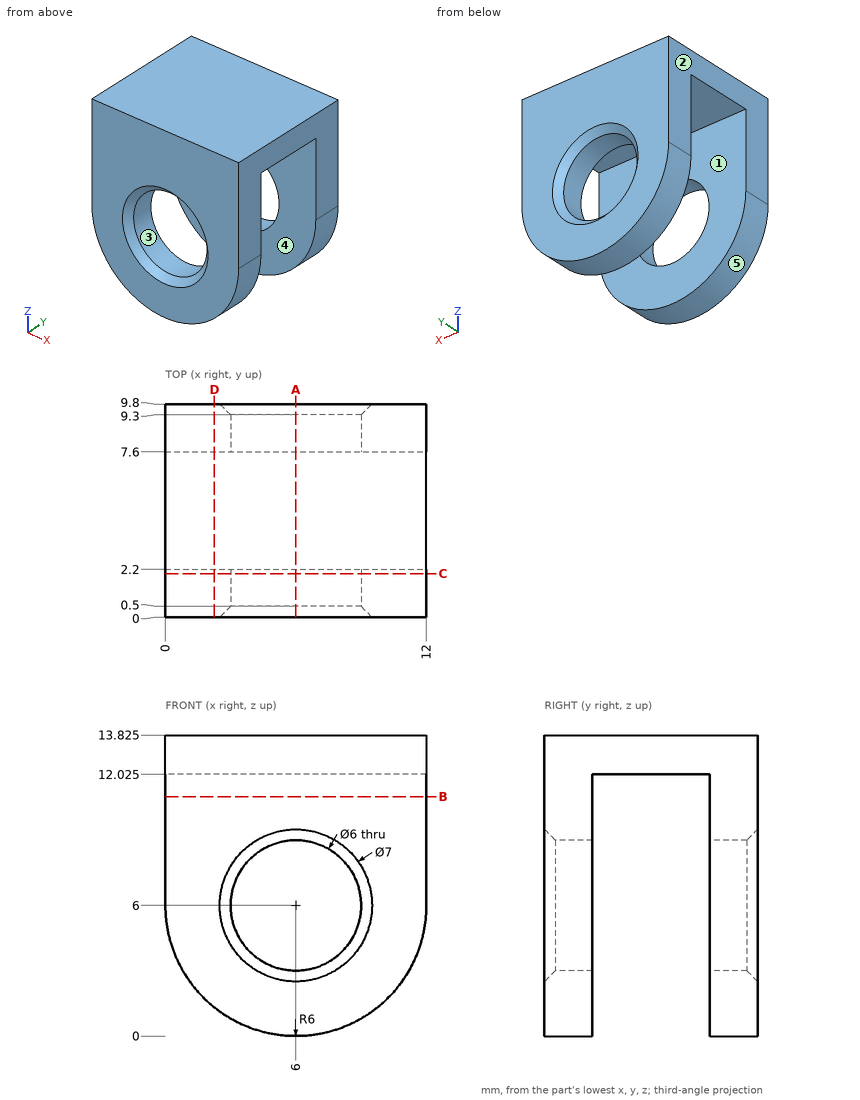
Geometry check sheet. Reference: drawing and pictorial views, mm from the part's lowest x, y, z. A direction names the side the tool comes from. Give positions to 0.01 mm unless a question says otherwise; leave off trailing zeros. Order: outer loops, then holes, each group sorted by start corner. A loop starts at its lowest first (then second) coordinate and runs counter-clockwise, first axis right, second up. Notation, with made-up numbers: M 53,-6 L 82,-6 A25 cw 82,14 Z; hole C 18,78 d8. An arc over 180 degrees is marked long. Use one line per item in the form item = value. Start each with the question number.
Q1. Scan lines: line 1 along Y through (x, z) = (9.25, 2.5); line 2 along X through (y, z) = (8.5, 6); line 3 along Z through (x, y) = (6, 8.75) (3 decimals). Record each from-to range of solid material in increasing order. Write a range as [from, to].
Q2. Access from +Z, -Z, +X, -X, +Y, -Y to the whole of each face (thin tool, end or side, straight path). Record for the marked faces 4 and 5.
Q3. Section check D-D (x = 2.25). Enter the section's corners in (y, z) (3 decimals).
Q4. Go/stop test with flat-tipped pins: pin 1 Ø1.5 at (y, z) = (2, 5) entering from -X; pin 2 Ø4 at (x, y) = (3.5, 3.5) entering from -Z; pin 3 Ø1 at (x, y) = (8.5, 8) entering from -Z. Record where each tip stops, or that it passes through.
Q5. Section check A-A (x = 6). Enter the section's corners in (y, z) (3 decimals).
Q6. Section check C-C (y = 2). Enter the section's corners in (x, z) (3 decimals).
Q7. Mould release check, pull along X, two halves, no side actions. Record for the marked faces 1, 2 and 3: +X half, -X half, draft (parallel to the pull), parting line (faces both ways), or undercut.
Q8. Section check B-B (z = 11). Enter the section's corners in (x, y).
Evaluation:
q1.line_1 = [0, 2.2], [7.6, 9.8]
q1.line_2 = [0, 3], [9, 12]
q1.line_3 = [0, 3], [9, 13.825]
q2.face_4 = -Z, +X, -X
q2.face_5 = -Z, +Y, -Y
q3.outline = M 0,1.316 L 2.2,1.316 L 2.2,12.025 L 7.6,12.025 L 7.6,1.316 L 9.8,1.316 L 9.8,13.825 L 0,13.825 Z
q4.pin_1 = 0.01
q4.pin_2 = 0.08
q4.pin_3 = 0.34
q5.outline = M 0,0 L 2.2,0 L 2.2,3 L 0.5,3 L 0,2.5 Z; M 0,9.5 L 0.5,9 L 2.2,9 L 2.2,12.025 L 7.6,12.025 L 7.6,9 L 9.3,9 L 9.8,9.5 L 9.8,13.825 L 0,13.825 Z; M 7.6,0 L 9.8,0 L 9.8,2.5 L 9.3,3 L 7.6,3 Z
q6.outline = M 0,6 A6 ccw 12,6 L 12,13.825 L 0,13.825 Z; hole C 6,6 d6
q7.face_1 = draft
q7.face_2 = -X half
q7.face_3 = undercut
q8.outline = M 0,0 L 12,0 L 12,2.2 L 0,2.2 Z; M 0,7.6 L 12,7.6 L 12,9.8 L 0,9.8 Z
